Can you work these out from the drawing? Everything is in mm from the part's minimum corner. A direction names the side the tool comes from. Round coordinates to 2 decimals unless told otherwise and drop trailing zeros. Write each loop counter-clockwise with the first axis right and the second up, starting at its lowest first coordinate (ties: lowest second). Pieces come first, ordered by that corner, then holes. Notation, with made-up numbers: M 76,-1 L 122,-1 A22 ccw 122,26 Z; hole C 1.5,24 d3. An arc over 180 degrees is marked long. Use a Markdown table: item, result. Add a question column.
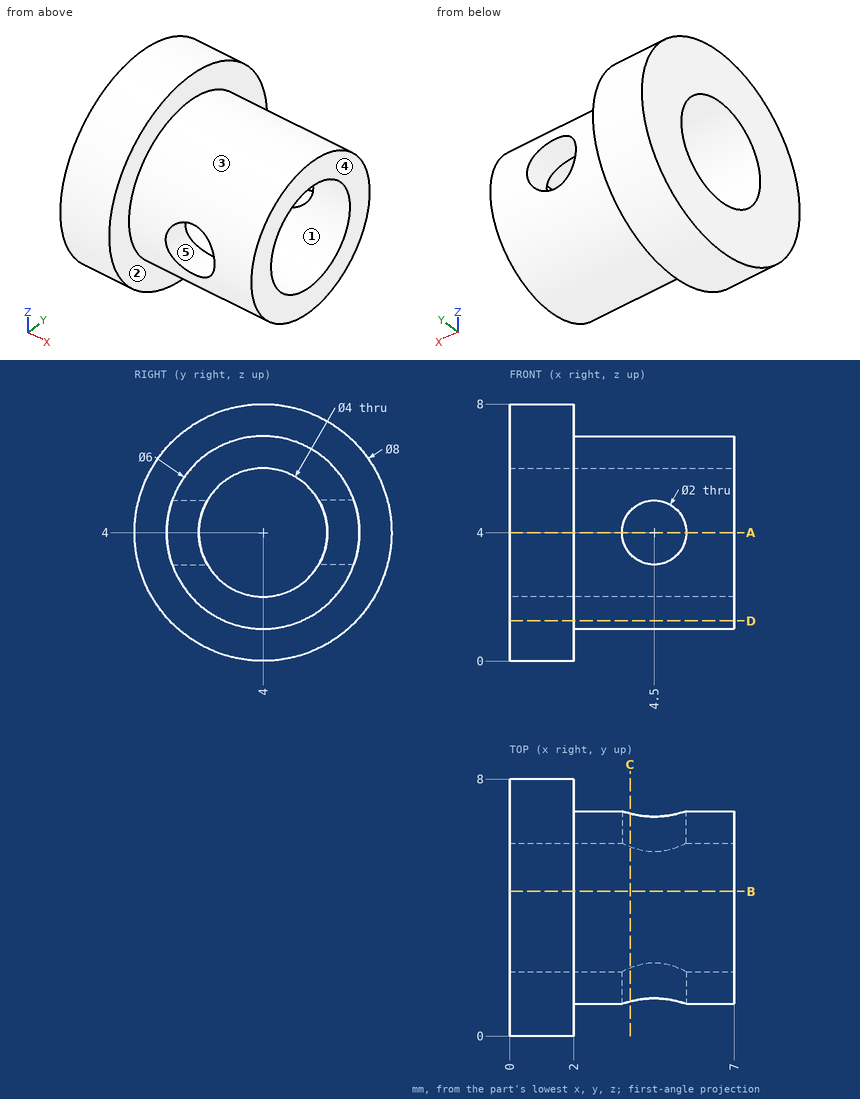
Item 1: On a 3-axis mill with a long thin cutter (end or side, diameter ignored), from which of +Z, -Z, +X, -X, +Y, -Y can I reach the whole of each face in a straight line? I mean the marked faces 1 and 2. Say none if no direction works.
Item 2: If we mould it in two halves opening along Z, with no side actions, what happens to the marked faces 3, 4 and 5? For each: +Z half, -Z half, draft (parallel to the pull), parting line (faces both ways), or undercut.
Item 3: Imagine slicing it at B-B on y = 4.5. List the corners of the cut face in (x, z) for me, plus the area to 3 significant figures.
Item 4: Imagine slicing it at D-D on z = 1.25. List the corners of the cut face in (x, y) for me.
Item 5: I need wall thicknesses on probe 1 along X at (y, z) = (6.6, 4); probe 2 along Y at (x, z) = (3.25, 4); probe 3 along X at (y, z) = (2, 6.75). Which ranges of each line are inside material? Lowest first, please. Write a range as from..to.
Item 6: Imagine slicing it at C-C on x = 3.75. List the corners of the cut face in (y, z) for me.
Item 7: Imagine slicing it at A-A on z = 4. List the corners of the cut face in (x, y) for me.
Item 8: For pin 1 Ø4 at (x, y) = (4.5, 2) entering from +Z; pin 2 Ø4 at (x, z) = (6.5, 3.5) entering from +Y; pin 3 Ø1.2 at (x, z) = (4.5, 4) entering from +Y; pin 4 Ø1 at (x, y) = (4.5, 2.5) entering from -Z, each with a flat end and sliding along its axis, tell me the tip position at first contact or that it passes through.
The answers:
| question | item | result |
|---|---|---|
| 1 | face 1 | +X, -X |
| 1 | face 2 | +X |
| 2 | face 3 | parting line |
| 2 | face 4 | draft |
| 2 | face 5 | undercut |
| 3 | outline | M 0,0.03 L 2,0.03 L 2,1.04 L 7,1.04 L 7,2.06 L 0,2.06 Z; M 0,5.94 L 7,5.94 L 7,6.96 L 2,6.96 L 2,7.97 L 0,7.97 Z |
| 3 | area | 18.3 mm² |
| 4 | outline | M 0,1.1 L 2,1.1 L 2,2.8 L 7,2.8 L 7,5.2 L 2,5.2 L 2,6.9 L 0,6.9 Z |
| 5 | probe 1 | 0..3.5, 5.5..7 |
| 5 | probe 2 | 1..2, 6..7 |
| 5 | probe 3 | 0..2 |
| 6 | outline | M 1.07,3.34 A3 ccw 6.93,3.34 L 5.89,3.34 A2 cw 2.11,3.34 Z; M 1.07,4.66 L 2.11,4.66 A2 cw 5.89,4.66 L 6.93,4.66 A3 ccw Z |
| 7 | outline | M 0,0 L 2,0 L 2,1 L 3.5,1 L 3.5,2 L 0,2 Z; M 0,6 L 3.5,6 L 3.5,7 L 2,7 L 2,8 L 0,8 Z; M 5.5,1 L 7,1 L 7,2 L 5.5,2 Z; M 5.5,6 L 7,6 L 7,7 L 5.5,7 Z |
| 8 | pin 1 | z = 7 |
| 8 | pin 2 | y = 7 |
| 8 | pin 3 | through |
| 8 | pin 4 | z = 1.17 |
